Could you check a few things on this model? Use its own coordinates, in mm. A direction names the side the tool comes from. Give positions to 0.01 mm unless a question says otherwise; leave off trailing zeros. Order: outer loops, then holes, each group sorted by start corner. A loop starts at its lowest first (then second) coordinate and runs counter-clockwise, first axis right, second up. Notation, with made-up numbers: (14.25, -31) -> (58.25, -31) arc R33 cw to (58.25, 3) -> close; hole circle Ø2 at (85, -23). An arc over 180 degrees is marked (long way). Answer as CSV lines item,"result". Start each with the question number.
(1) I need wall thicknesses on L1, parallel to X at y = -3.5, z = 5.5; L2, parallel to Z at x = 2.25, y = -0.25; L3, parallel to Z at x = 5.25, y = -2.5. Which ranges of each line are inside material? Lowest first, please.
(2) I want a section at D-D (x = 8.5). Please give me the cut outline in (y, z).
(3) I want a section at A-A (z = 5.6). Please give me the cut outline in (x, y).
(4) I want a section at C-C (y = -4.5). Please give me the cut outline in (x, z).
(5) On a 3-axis mill with a long thin cutter (end or side, diameter ignored), from which of +Z, -Z, +X, -X, +Y, -Y can I reach the whole of each face in a straight line? I mean faces 5 (the face through (3.7, -1.6, 9.6)), 6 (the face through (1.493, -3, 5)). Say none if no direction works.
(6) I want a section at B-B (x = 4.5). Please give me the cut outline in (y, z).
(7) We'd pull the mould along X, two halves only. Please class faces 1 (the face through (7.71, -4.35, 10.39)), 2 (the face through (9.493, -3, 5)), 3 (the face through (5, -3, 11.2)), 4 (the face through (7.71, -3.49, 4.68)): released by +X, released by -X, zero draft, split by the parting line, or undercut.
```python
from build123d import *

# Parameters (mm, degrees)
F0_W     = 8
F0_H     = 8
F1_DEPTH = 9.6
F2_R     = 2.4
F3_DEPTH = 25
F4_R     = 2.4
F5_DEPTH = 1.6


with BuildPart() as f1:
    # F0 (on Top) → F1 (new body)
    with BuildSketch(Plane.XY):
        with Locations((5.493415, -3.433774)):
            Rectangle(F0_W, F0_H)
    extrude(amount=F1_DEPTH)

    # F2 (on face) → F3 (cut)
    with BuildSketch(Plane.XZ.offset(7.433774)):
        with Locations((5.493415, 5.6)):
            Circle(F2_R)
    extrude(amount=-F3_DEPTH, mode=Mode.SUBTRACT)

    # F4 (on face) → F5 (join)
    with BuildSketch(Plane.XY.offset(9.6)):
        with Locations((5.493415, -3.433774)):
            Circle(F4_R)
    extrude(amount=F5_DEPTH)


solid = f1.part
```
Final values:
1,L1,"1.49 to 3.1, 7.89 to 9.49"
1,L2,"0 to 9.6"
1,L3,"0 to 3.21, 7.99 to 11.2"
2,outline,"(-7.43, 0) -> (0.57, 0) -> (0.57, 9.6) -> (-7.43, 9.6) -> close"
3,outline,"(1.49, -7.43) -> (3.09, -7.43) -> (3.09, 0.57) -> (1.49, 0.57) -> close; (7.89, -7.43) -> (9.49, -7.43) -> (9.49, 0.57) -> (7.89, 0.57) -> close"
4,outline,"(1.49, 0) -> (9.49, 0) -> (9.49, 9.6) -> (7.64, 9.6) -> (7.64, 11.2) -> (3.34, 11.2) -> (3.34, 9.6) -> (1.49, 9.6) -> close; hole circle Ø4.8 at (5.49, 5.6)"
5,face 5,"+Z"
5,face 6,"+Z, -Z, -X, +Y, -Y"
6,outline,"(-7.43, 0) -> (0.57, 0) -> (0.57, 3.42) -> (-7.43, 3.42) -> close; (-7.43, 7.78) -> (0.57, 7.78) -> (0.57, 9.6) -> (-1.25, 9.6) -> (-1.25, 11.2) -> (-5.62, 11.2) -> (-5.62, 9.6) -> (-7.43, 9.6) -> close"
7,face 1,"split by the parting line"
7,face 2,"released by +X"
7,face 3,"zero draft"
7,face 4,"undercut"
